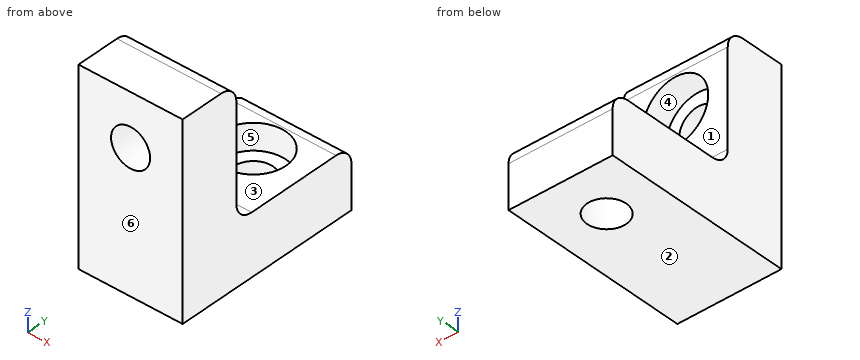
```python
from build123d import *

# Parameters (mm, degrees)
SKETCH_W        = 12
SKETCH_H        = 22
PAD_DEPTH       = 7
SKETCH001_W     = 12
SKETCH001_H     = 7
PAD001_DEPTH    = 15
SKETCH002_R     = 2.25
POCKET_DEPTH    = 10
SKETCH003_R     = 3.75
POCKET001_DEPTH = 3
SKETCH004_R     = 2.25
POCKET002_DEPTH = 7
SKETCH005_R     = 3.75
POCKET003_DEPTH = 3
FILLET_R        = 2


with BuildPart() as part:
    # Sketch → Pad (new body)
    with BuildSketch(Plane.XY):
        with Locations((0, 11)):
            Rectangle(SKETCH_W, SKETCH_H)
    extrude(amount=PAD_DEPTH)

    # Sketch001 (on Face6 of Pad) → Pad001 (join)
    with BuildSketch(Plane.XY.offset(7)):
        with Locations((0, 3.5)):
            Rectangle(SKETCH001_W, SKETCH001_H)
    extrude(amount=PAD001_DEPTH)

    # Sketch002 (on Face3 of Pad001) → Pocket (cut)
    with BuildSketch(Plane.XY.offset(7)):
        with Locations((0, 16)):
            Circle(SKETCH002_R)
    extrude(amount=-POCKET_DEPTH, mode=Mode.SUBTRACT)

    # Sketch003 (on Face9 of Pocket) → Pocket001 (cut)
    with BuildSketch(Plane.XY.offset(7)):
        with Locations((0, 16)):
            Circle(SKETCH003_R)
    extrude(amount=-POCKET001_DEPTH, mode=Mode.SUBTRACT)

    # Sketch004 (on Face8 of Pocket001) → Pocket002 (cut)
    with BuildSketch(Plane(origin=(0, 7, 0), x_dir=(-1, 0, 0), z_dir=(0, 1, 0))):
        with Locations((0, 16)):
            Circle(SKETCH004_R)
    extrude(amount=-POCKET002_DEPTH, mode=Mode.SUBTRACT)

    # Sketch005 (on Face9 of Pocket002) → Pocket003 (cut)
    with BuildSketch(Plane(origin=(0, 7, 0), x_dir=(-1, 0, 0), z_dir=(0, 1, 0))):
        with Locations((0, 16)):
            Circle(SKETCH005_R)
    extrude(amount=-POCKET003_DEPTH, mode=Mode.SUBTRACT)

    # Fillet
    fillet_edges = [part.edges().sort_by_distance(p)[0] for p in [
        (0, 7, 7),
        (0, 7, 22),
        (0, 22, 7),
    ]]
    fillet(fillet_edges, radius=FILLET_R)


solid = part.part
```
Model file for the job. Use its own axes, mm. Face numbers are marked on the shaded views. A direction names the side the tool comes from. Give positions to 0.01 mm unless a question says otherwise; leave off trailing zeros. Loops run counter-clockwise (first coordinate to the right, second up) from the corner with the lowest first, then second, coordinate; pieces in that order, holes last. Notation, with made-up numbers: (6, -16.5) -> (41, -16.5) arc R16 cw to (41, 14.5) -> close; hole circle Ø10 at (73, 10.5). An arc over 180 degrees is marked (long way). Use CSV: the item, a comma, the result in double quotes. Start each with the question number.
1) Mould opens along Z. For the marked faces 1, 2, 3 and 4 say: released by +Z, released by -Z, zero draft, split by the parting line, or undercut.
2) Wall check: line 1 (Y direction, x = 0, z = 4.75); line 2 (X direction, y = 13, z = 5.5); line 3 (Y direction, x = 0, z = 1.35). Give the ranges that are in metal, low to high.
3) Slice it at C-C on y = 16.5. Give the cut face in (x, z), plus the area to 3 significant figures.
4) Slice it at D-D on z = 3.5. Give the cut face in (x, y).
5) Slice it at B-B on z = 16. Give the cut face in (x, y), plus the area to 3 significant figures.
6) Slice it at A-A on x = 0. Give the cut face in (y, z).
7) Flat gauge pins, fed straight in: pin 1 Ø5.5 at (x, z) = (1, 12) entering from +Y; pin 2 Ø6 at (y, z) = (12, 12.5) entering from +X; pin 3 Ø5 at (x, y) = (0, 16) entering from +Z; pin 4 Ø4 at (x, y) = (-2, 14) entering from +Z. Where does each tip first touch, or does it go through?
8) Tool access for the marked faces 5 and 6: list every direction of +Z, -Z, +X, -X, +Y, -Y with a clear straight run to the whole face (end or side of a thin tool).
Computed values:
1,face 1,"zero draft"
1,face 2,"released by -Z"
1,face 3,"released by +Z"
1,face 4,"undercut"
2,line 1,"y = 0 to 12.25, 19.75 to 22"
2,line 2,"x = -6 to -2.25, 2.25 to 6"
2,line 3,"y = 0 to 13.75, 18.25 to 22"
3,outline,"(-6, 0) -> (-2.19, 0) -> (-2.19, 4) -> (-3.72, 4) -> (-3.72, 7) -> (-6, 7) -> close; (2.19, 0) -> (6, 0) -> (6, 7) -> (3.72, 7) -> (3.72, 4) -> (2.19, 4) -> close"
3,area,"44.2 mm^2"
4,outline,"(-6, 0) -> (6, 0) -> (6, 22) -> (-6, 22) -> close; hole circle Ø4.5 at (0, 16)"
5,outline,"(-6, 0) -> (-2.25, 0) -> (-2.25, 4) -> (-3.75, 4) -> (-3.75, 7) -> (-6, 7) -> close; (2.25, 0) -> (6, 0) -> (6, 7) -> (3.75, 7) -> (3.75, 4) -> (2.25, 4) -> close"
5,area,"43.5 mm^2"
6,outline,"(0, 0) -> (13.75, 0) -> (13.75, 4) -> (12.25, 4) -> (12.25, 7) -> (9, 7) arc R2 cw to (7, 9) -> (7, 12.25) -> (4, 12.25) -> (4, 13.75) -> (0, 13.75) -> close; (0, 18.25) -> (4, 18.25) -> (4, 19.75) -> (7, 19.75) -> (7, 20) arc R2 ccw to (5, 22) -> (0, 22) -> close; (18.25, 0) -> (22, 0) -> (22, 5) arc R2 ccw to (20, 7) -> (19.75, 7) -> (19.75, 4) -> (18.25, 4) -> close"
7,pin 1,"stops at y = 7"
7,pin 2,"passes through"
7,pin 3,"stops at z = 4"
7,pin 4,"stops at z = 7"
8,face 5,"+Z"
8,face 6,"+Z, -Z, +X, -X, -Y"
